from build123d import *

# Parameters (mm, degrees)
BOSS_EXTRUDE1_DEPTH                             = 132
CSK_FOR_M3_FLAT_HEAD_MACHINE_SCREW1_D           = 3.4
CSK_FOR_M3_FLAT_HEAD_MACHINE_SCREW1_DEPTH       = 5
CSK_FOR_M3_FLAT_HEAD_MACHINE_SCREW1_CSINK_D     = 6.3
CSK_FOR_M3_FLAT_HEAD_MACHINE_SCREW1_CSINK_ANGLE = 90
CSK_FOR_M3_FLAT_HEAD_MACHINE_SCREW1_TIP         = 1.021463052
CSK_FOR_M3_FLAT_HEAD_MACHINE_SCREW2_D           = 3.4
CSK_FOR_M3_FLAT_HEAD_MACHINE_SCREW2_DEPTH       = 5
CSK_FOR_M3_FLAT_HEAD_MACHINE_SCREW2_CSINK_D     = 6.3
CSK_FOR_M3_FLAT_HEAD_MACHINE_SCREW2_CSINK_ANGLE = 90
CSK_FOR_M3_FLAT_HEAD_MACHINE_SCREW2_TIP         = 1.021463052
CUT_EXTRUDE1_DEPTH                              = 5
LPATTERN1_COUNT                                 = 17
LPATTERN1_PITCH                                 = 6
CUT_EXTRUDE2_DEPTH                              = 200
LPATTERN2_COUNT                                 = 10
LPATTERN2_PITCH                                 = 6
FILLET1_R                                       = 4


with BuildPart() as part:
    # Sketch1 → Boss-Extrude1 (new body)
    with BuildSketch(Plane.XY):
        with BuildLine():
            Line((0, 0), (-2, 0))
            Line((-2, 0), (-2, 54.2))
            ThreePointArc((-2, 54.2), (-1.472792206, 55.472792206), (-0.2, 56))
            Line((-0.2, 56), (285.2, 56))
            ThreePointArc((285.2, 56), (286.472792206, 55.472792206), (287, 54.2))
            Line((287, 54.2), (287, 0))
            Line((287, 0), (285, 0))
            Line((285, 0), (285, 53.5))
            ThreePointArc((285, 53.5), (284.853553391, 53.853553391), (284.5, 54))
            Line((284.5, 54), (0.5, 54))
            ThreePointArc((0.5, 54), (0.146446609, 53.853553391), (0, 53.5))
            Line((0, 53.5), (0, 0))
        make_face()
    extrude(amount=BOSS_EXTRUDE1_DEPTH)

    # CSK for M3 Flat Head Machine Screw1
    with Locations(Plane.ZY.offset(2)):
        with Locations((8.5, 45), (8.5, 15), (123.5, 45), (123.5, 15)):
            CounterSinkHole(CSK_FOR_M3_FLAT_HEAD_MACHINE_SCREW1_D / 2, CSK_FOR_M3_FLAT_HEAD_MACHINE_SCREW1_CSINK_D / 2, depth=CSK_FOR_M3_FLAT_HEAD_MACHINE_SCREW1_DEPTH, counter_sink_angle=CSK_FOR_M3_FLAT_HEAD_MACHINE_SCREW1_CSINK_ANGLE)
            with Locations((0, 0, -(CSK_FOR_M3_FLAT_HEAD_MACHINE_SCREW1_DEPTH + CSK_FOR_M3_FLAT_HEAD_MACHINE_SCREW1_TIP / 2))):  # 118° drill point
                Cone(0, CSK_FOR_M3_FLAT_HEAD_MACHINE_SCREW1_D / 2, CSK_FOR_M3_FLAT_HEAD_MACHINE_SCREW1_TIP, mode=Mode.SUBTRACT)

    # CSK for M3 Flat Head Machine Screw2
    with Locations(Plane(origin=(287, 0, 0), x_dir=(0, 0, -1), z_dir=(1, 0, 0))):
        with Locations((-123.5, 45), (-123.5, 15), (-8.5, 45), (-8.5, 15)):
            CounterSinkHole(CSK_FOR_M3_FLAT_HEAD_MACHINE_SCREW2_D / 2, CSK_FOR_M3_FLAT_HEAD_MACHINE_SCREW2_CSINK_D / 2, depth=CSK_FOR_M3_FLAT_HEAD_MACHINE_SCREW2_DEPTH, counter_sink_angle=CSK_FOR_M3_FLAT_HEAD_MACHINE_SCREW2_CSINK_ANGLE)
            with Locations((0, 0, -(CSK_FOR_M3_FLAT_HEAD_MACHINE_SCREW2_DEPTH + CSK_FOR_M3_FLAT_HEAD_MACHINE_SCREW2_TIP / 2))):  # 118° drill point
                Cone(0, CSK_FOR_M3_FLAT_HEAD_MACHINE_SCREW2_D / 2, CSK_FOR_M3_FLAT_HEAD_MACHINE_SCREW2_TIP, mode=Mode.SUBTRACT)

    # Sketch6 → Cut-Extrude1 (cut)
    with BuildSketch(Plane(origin=(0, 56, 0), x_dir=(1, 0, 0), z_dir=(0, 1, 0))):
        with BuildLine():
            Line((67.2, -13), (142.2, -13))
            ThreePointArc((142.2, -13), (144.2, -15), (142.2, -17))
            Line((142.2, -17), (67.2, -17))
            ThreePointArc((67.2, -17), (65.2, -15), (67.2, -13))
        make_face()
    cut_extrude1 = extrude(amount=-CUT_EXTRUDE1_DEPTH, mode=Mode.SUBTRACT)

    # LPattern1: Cut-Extrude1 ×17
    with Locations(*[(0, 0, i * LPATTERN1_PITCH) for i in range(1, LPATTERN1_COUNT)]):
        add(cut_extrude1, mode=Mode.SUBTRACT)

    # Sketch7 → Cut-Extrude2 (cut)
    with BuildSketch(Plane(origin=(0, 56, 0), x_dir=(1, 0, 0), z_dir=(0, 1, 0))):
        with BuildLine():
            Line((205.2, -13), (270.2, -13))
            ThreePointArc((270.2, -13), (272.2, -15), (270.2, -17))
            Line((270.2, -17), (205.2, -17))
            ThreePointArc((205.2, -17), (203.2, -15), (205.2, -13))
        make_face()
    cut_extrude2 = extrude(amount=-CUT_EXTRUDE2_DEPTH, mode=Mode.SUBTRACT)

    # LPattern2: Cut-Extrude2 ×10
    with Locations(*[(0, 0, i * LPATTERN2_PITCH) for i in range(1, LPATTERN2_COUNT)]):
        add(cut_extrude2, mode=Mode.SUBTRACT)

    # Fillet1
    fillet1_edges = [part.edges().sort_by_distance(p)[0] for p in [
        (-1, 0, 0),
        (286, 0, 0),
        (286, 0, 132),
        (-1, 0, 132),
    ]]
    fillet(fillet1_edges, radius=FILLET1_R)


solid = part.part
For this review, take the finished solid that the model builds, in its own axes (mm). A direction names the side the tool comes from. Round coordinates to 2 decimals unless told otherwise and drop trailing zeros. Order: outer loops, then holes, each group sorted by start corner. A loop starts at its lowest first (then second) coordinate and runs counter-clockwise, first axis right, second up. Notation, with made-up numbers: (66.25, 74.5) -> (77.25, 74.5) arc R9 cw to (77.25, 83.5) -> close; hole circle Ø4 at (23.5, 22.25). An arc over 180 degrees is marked (long way). Write item = value, one per line. Start each with the question number.
1) Tool access review of faces 1 (the face through (143, 55, 132)), 2 (the face through (285, 26, 65)): name each direction out of +Z, -Z, +X, -X, +Y, -Y from which nothing blocks a thin tool from reaching the whole face with its end or side.
2) Take a section at A-A on y = 22.5. State the section outline as (x, z) points.
3) Take a section at C-C on z = 117.5. State the section outline as (x, y) points, plus the area to 3 significant figures.
4) Insertion check: pin 1 (2 mm diameter, centred on x = 51, z = 42, fed in from -Y). The pin has a flat end and moves straight along its axis. Give the tip position at first contact, or say it passes through.
5) Take a section at B-B on x = 102. Count the separate pieces of the cut face and the enclosed holes in it, plus the area to 3 significant figures.
6) To check wall thickness, follow line 1 (Y direction, x = -0.25, z = 123.5); line 2 (Z direction, x = 285.4, y = 15); line 3 (X direction, y = 20.5, z = 92.5). State the ranges of each line that lie inside material, in increasing order. Write a range as from..to.
Verdict:
q1.face_1 = +Z, +X, -X, +Y, -Y
q1.face_2 = +Z, -Z, -Y
q2.outline = (-2, 0) -> (0, 0) -> (0, 132) -> (-2, 132) -> close; (285, 0) -> (287, 0) -> (287, 132) -> (285, 132) -> close
q3.outline = (-2, 0) -> (0, 0) -> (0, 53.5) arc R0.5 cw to (0.5, 54) -> (284.5, 54) arc R0.5 cw to (285, 53.5) -> (285, 0) -> (287, 0) -> (287, 54.2) arc R1.8 ccw to (285.2, 56) -> (-0.2, 56) arc R1.8 ccw to (-2, 54.2) -> close
q3.area = 793 mm2
q4.pin_1 = 54
q5.separate_pieces = 18
q5.enclosed_holes = 0
q5.area = 128 mm2
q6.line_1 = 0..13.3, 16.7..43.3, 46.7..56
q6.line_2 = 0..6.8, 10.2..121.8, 125.2..132
q6.line_3 = -2..0, 285..287
